Geometry check sheet. Reference: the model listing, model coordinates, mm. Face numbers are marked on the shaded views. Round coordinates to 2 decimals unless told otherwise and drop trailing zeros. Order: outer loops, then holes, each group sorted by start corner. A loop starts at its lowest first (then second) coordinate and runs counter-clockwise, first axis right, second up.
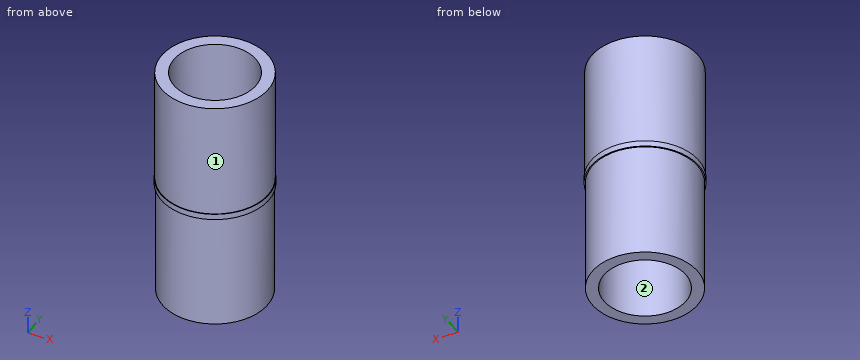
```python
from build123d import *

# Parameters (mm, degrees)
F0_R     = 9.25
F1_DEPTH = 1
F2_R     = 9.15
F3_DEPTH = 20
F4_R     = 9.05
F5_DEPTH = 20
F6_R     = 7.05
F7_DEPTH = 41.001


with BuildPart() as f1:
    # F0 (on Top) → F1 (new body)
    with BuildSketch(Plane.XY):
        Circle(F0_R)
    extrude(amount=F1_DEPTH)

    # F2 (on face) → F3 (join)
    with BuildSketch(Plane.XY.offset(1)):
        Circle(F2_R)
    extrude(amount=F3_DEPTH)

    # F4 (on face) → F5 (join)
    with BuildSketch(Plane(origin=(0, 0, 0), x_dir=(1, 0, 0), z_dir=(0, 0, -1))):
        Circle(F4_R)
    extrude(amount=F5_DEPTH)

    # F6 (on face) → F7 (cut, through all)
    with BuildSketch(Plane(origin=(0, 0, -20), x_dir=(1, 0, 0), z_dir=(0, 0, -1))):
        Circle(F6_R)
    extrude(amount=-F7_DEPTH, mode=Mode.SUBTRACT)


solid = f1.part
```
(1) Depth check by flat-ended pin: P1, Ø3, axis at x = -5, z = 6.5, coming from the +Y side; P2, Ø2, axis at x = 4, y = -3.5, coming from the +Z side; P3, Ø6, axis at y = 4, z = 3, coming from the +X side; P4, Ø3, axis at y = -4.5, z = -1, coming from the +X side. Enter the tip coordinate at first touch or a pass-through.
Returned:
P1: stops at y = 8.45
P2: passes through
P3: stops at x = 9.1
P4: stops at x = 8.61
(2) Sectioned sample at D-D, the plane x = 8.25. Record the cut outline in (y, z).
Returned:
outline: (-4.18, 0) - (-3.72, 0) - (-3.72, -20) - (3.72, -20) - (3.72, 0) - (4.18, 0) - (4.18, 1) - (3.96, 1) - (3.96, 21) - (-3.96, 21) - (-3.96, 1) - (-4.18, 1) - close
(3) Draft check along X on the marked faces 1 and 2. Enter one of: released by +X, released by -X, zero draft, split by the parting line, or undercut.
Returned:
face 1: split by the parting line
face 2: undercut
(4) Sectioned sample at A-A, the plane x = 0. Record the cut outline in (y, z), and give its area (3 significant figures).
Returned:
outline: (-9.25, 0) - (-9.05, 0) - (-9.05, -20) - (-7.05, -20) - (-7.05, 21) - (-9.15, 21) - (-9.15, 1) - (-9.25, 1) - close; (7.05, -20) - (9.05, -20) - (9.05, 0) - (9.25, 0) - (9.25, 1) - (9.15, 1) - (9.15, 21) - (7.05, 21) - close
area: 168 mm2
(5) Material ranges on line 1 (Y direction, x = 0, z = 9); line 2 (X direction, y = 0, z = -2.5); line 3 (Y direction, x = -4, z = -3), recorded low to high.
Returned:
line 1: y = -9.15 to -7.05, 7.05 to 9.15
line 2: x = -9.05 to -7.05, 7.05 to 9.05
line 3: y = -8.12 to -5.81, 5.81 to 8.12
(6) Sectioned sample at C-C, the plane z = 17.5. Record the cut outline in (x, y), and give its area (3 significant figures).
Returned:
outline: circle Ø18.3 at (0, 0); hole circle Ø14.1 at (0, 0)
area: 107 mm2
